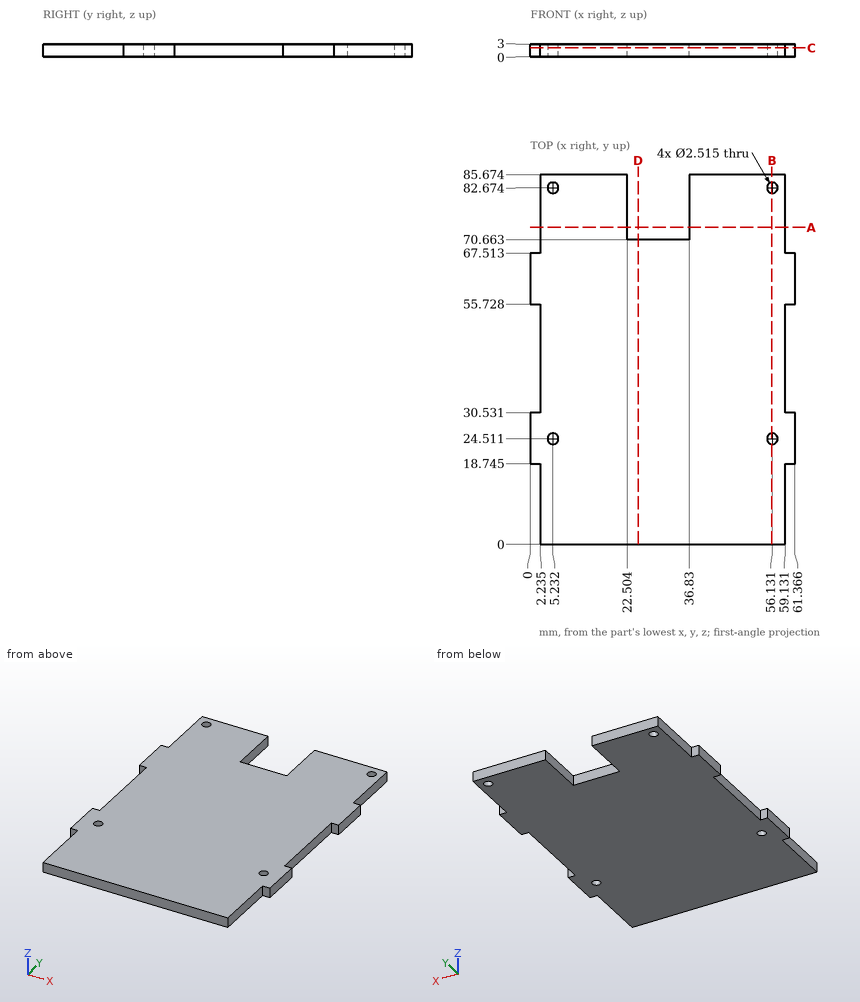
Geometry: see drawing. Coordinates: mm, zero at the bounding-box minimum. Give positions to 0.01 mm unless a question says otherwise; leave off trailing zeros. Order: outer loops, then holes, each group sorted by start corner. A loop starts at its lowest first (then second) coordinate and runs counter-clockwise, first axis right, second up. Notation, with made-up numbers: (-25.5, -18.75) - (29.5, -18.75) arc R21 ccw to (29.5, -14.75) - close; hole circle Ø2 at (-27, -0.75). An arc over 180 degrees is marked (long way). One line per item, written item: value.
1. Cut plane B-B, the plane x = 56. Output: boundary loops of the cut face in (y, z) (1 decimal), and give its area (3 significant figures).
Determined:
outline: (0, 0) - (23.3, 0) - (23.3, 3) - (0, 3) - close; (25.8, 0) - (81.4, 0) - (81.4, 3) - (25.8, 3) - close; (83.9, 0) - (85.7, 0) - (85.7, 3) - (83.9, 3) - close
area: 242 mm2
2. Line query: probe 1 along Y at (x, z) = (56, 1.75) (1 decimal); probe 2 along X at (y, z) = (75.5, 1.8) (1 decimal); probe 3 along X at (y, z) = (45, 0.9) (1 decimal). Output: solid intervals per line, ascending.
Determined:
probe 1: 0 to 23.3, 25.8 to 81.4, 83.9 to 85.7
probe 2: 2.2 to 22.5, 36.8 to 59.1
probe 3: 2.2 to 59.1
3. Cut plane D-D, the plane x = 25. Output: boundary loops of the cut face in (y, z).
Determined:
outline: (0, 0) - (70.66, 0) - (70.66, 3) - (0, 3) - close
4. Pin query (flat end, axial travel): pin 1 Ø1.1 at (x, z) = (1.5, 1.5) entering from +Y; pin 2 Ø1.5 at (y, z) = (12.5, 1) entering from +X; pin 3 Ø1.1 at (x, z) = (60, 1.5) entering from -Y (1 decimal); pin 4 Ø8 at (x, y) = (43.5, 54) entering from -Z. Return the tip coordinate at first contact, or that it passes through.
Determined:
pin 1: y = 67.51
pin 2: x = 59.13
pin 3: y = 18.7
pin 4: z = 0
5. Cut plane C-C, the plane z = 2.1. Output: boundary loops of the cut face in (x, y) (1 decimal).
Determined:
outline: (0, 18.7) - (2.2, 18.7) - (2.2, 0) - (59.1, 0) - (59.1, 18.7) - (61.4, 18.7) - (61.4, 30.5) - (59.1, 30.5) - (59.1, 55.7) - (61.4, 55.7) - (61.4, 67.5) - (59.1, 67.5) - (59.1, 85.7) - (36.8, 85.7) - (36.8, 70.7) - (22.5, 70.7) - (22.5, 85.7) - (2.2, 85.7) - (2.2, 67.5) - (0, 67.5) - (0, 55.7) - (2.2, 55.7) - (2.2, 30.5) - (0, 30.5) - close; hole circle Ø2.5 at (5.2, 24.5); hole circle Ø2.5 at (5.2, 82.7); hole circle Ø2.5 at (56.1, 24.5); hole circle Ø2.5 at (56.1, 82.7)
6. Cut plane A-A, the plane y = 73.5. Output: boundary loops of the cut face in (x, z) (1 decimal), and give its area (3 significant figures).
Determined:
outline: (2.2, 0) - (22.5, 0) - (22.5, 3) - (2.2, 3) - close; (36.8, 0) - (59.1, 0) - (59.1, 3) - (36.8, 3) - close
area: 128 mm2
